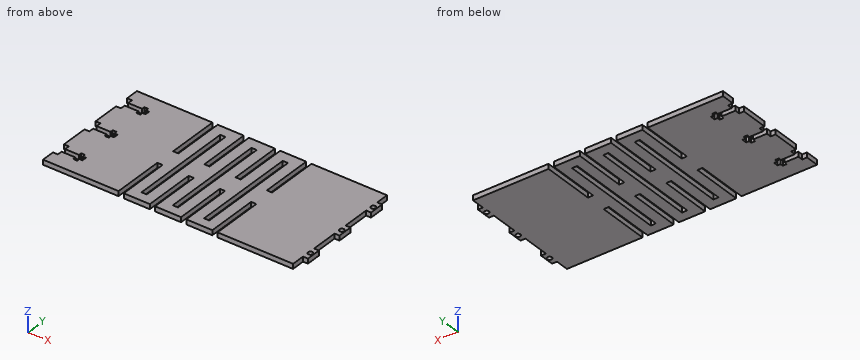
```python
from build123d import *

# Parameters (mm, degrees)
F0_W     = 3.175
F0_H     = 63.5
F0_R     = 1.4224
F1_DEPTH = 2.9718


with BuildPart() as f1:
    # F0 (on Top) → F1 (new body)
    with BuildSketch(Plane.XY):
        Polygon((0, 8.035559), (0, 0), (46.0375, 0), (46.0375, 31.32091), (49.2125, 31.32091), (49.2125, 0), (65.0875, 0), (65.0875, 31.32091), (68.2625, 31.32091), (68.2625, 0), (84.1375, 0), (84.1375, 31.32091), (87.3125, 31.32091), (87.3125, 0), (103.1875, 0), (103.1875, 31.32091), (106.3625, 31.32091), (106.3625, 0), (152.4, 0), (152.4, 8.035554), (155.3718, 8.035554), (155.3718, 11.058159), (155.3718, 13.902959), (155.3718, 16.925564), (152.4, 16.925564), (152.4, 33.489475), (155.3718, 33.489475), (155.3718, 36.51208), (155.3718, 39.35688), (155.3718, 42.379485), (152.4, 42.379485), (152.4, 58.943395), (155.3718, 58.943395), (155.3718, 61.966), (155.3718, 64.8108), (155.3718, 67.833405), (152.4, 67.833405), (152.4, 75.77091), (106.3625, 75.77091), (106.3625, 44.02091), (103.1875, 44.02091), (103.1875, 75.77091), (87.3125, 75.77091), (87.3125, 44.02091), (84.1375, 44.02091), (84.1375, 75.77091), (68.2625, 75.77091), (68.2625, 44.02091), (65.0875, 44.02091), (65.0875, 75.77091), (49.2125, 75.77091), (49.2125, 44.02091), (46.0375, 44.02091), (46.0375, 75.77091), (0, 75.77091), (0, 67.83341), (2.9718, 67.83341), (2.9718, 64.810805), (11.43, 64.810805), (11.43, 66.563405), (13.81125, 66.563405), (13.81125, 64.810805), (15.6718, 64.810805), (15.6718, 61.966005), (13.81125, 61.966005), (13.81125, 60.213405), (11.43, 60.213405), (11.43, 61.966005), (2.9718, 61.966005), (2.9718, 58.9434), (0, 58.9434), (0, 42.37949), (2.9718, 42.37949), (2.9718, 39.356885), (11.43, 39.356885), (11.43, 41.109485), (13.81125, 41.109485), (13.81125, 39.356885), (15.6718, 39.356885), (15.6718, 36.512085), (13.81125, 36.512085), (13.81125, 34.759485), (11.43, 34.759485), (11.43, 36.512085), (2.9718, 36.512085), (2.9718, 33.48948), (0, 33.48948), (0, 16.925569), (2.9718, 16.925569), (2.9718, 13.902964), (11.43, 13.902964), (11.43, 15.655564), (13.81125, 15.655564), (13.81125, 13.902964), (15.6718, 13.902964), (15.6718, 11.058164), (13.81125, 11.058164), (13.81125, 9.305564), (11.43, 9.305564), (11.43, 11.058164), (2.9718, 11.058164), (2.9718, 8.035559), align=None)
        with Locations((57.15, 37.67091)):
            Rectangle(F0_W, F0_H, mode=Mode.SUBTRACT)
        with Locations((76.2, 37.67091)):
            Rectangle(F0_W, F0_H, mode=Mode.SUBTRACT)
        with Locations((153.4668, 12.588405)):
            Circle(F0_R, mode=Mode.SUBTRACT)
        with Locations((95.25, 37.67091)):
            Rectangle(F0_W, F0_H, mode=Mode.SUBTRACT)
        with Locations((153.4668, 37.988405)):
            Circle(F0_R, mode=Mode.SUBTRACT)
        with Locations((153.4668, 63.388405)):
            Circle(F0_R, mode=Mode.SUBTRACT)
    extrude(amount=F1_DEPTH)


solid = f1.part
```
Source: CAD feature listing. Evaluate the final solid. Frame: model axes, mm. Give positions to 0.01 mm unless a question says otherwise; leave off trailing zeros. Put each result on its own line as item: value. Start each with the question number.
1) Material intervals for probe 1 along X at (y, z) = (41, 2.7); probe 2 along Y at (x, z) = (10, 1.15); probe 3 along Y at (x, z) = (12.5, 0.6), sorted ascending.
2) Cut plane A-A (y = 21). State how many separate pieces and enclosed holes the cut face has, then the cut area to 3 significant figures.
3) Contact query for flat-ended pins moving along their axis: P1, Ø1.5, axis at x = 1, z = 2, coming from the -Y side; P2, Ø1.5, axis at y = 11.5, z = 2, coming from the -X side. Output: stop coordinate, or through.
Results are:
1. probe 1: x = 2.97 to 11.43, 13.81 to 55.56, 58.74 to 74.61, 77.79 to 93.66, 96.84 to 155.37
1. probe 2: y = 0 to 11.06, 13.9 to 36.51, 39.36 to 61.97, 64.81 to 75.77
1. probe 3: y = 0 to 9.31, 15.66 to 34.76, 41.11 to 60.21, 66.56 to 75.77
2. separate pieces: 8
2. enclosed holes: 0
2. area: 387 mm2
3. P1: stops at y = 0
3. P2: stops at x = 2.97
